```python
from build123d import *

# Parameters (mm, degrees)
F0_R     = 225
F1_DEPTH = 60


with BuildPart() as f1:
    # F0 (on Front) → F1 (new body)
    with BuildSketch(Plane.XZ):
        with BuildLine():
            ThreePointArc((228.965063, -4), (228.991266, -2.000076), (229, 0))
            ThreePointArc((229, 0), (228.991266, 2.000076), (228.965063, 4))
            ThreePointArc((228.965063, 4), (0, 229), (-228.965063, 4))
            ThreePointArc((-228.965063, 4), (-229, 0), (-228.965063, -4))
            ThreePointArc((-228.965063, -4), (0, -229), (228.965063, -4))
        make_face()
        Circle(F0_R, mode=Mode.SUBTRACT)
        with BuildLine():
            ThreePointArc((228.965063, 4), (228.991266, 2.000076), (229, 0))
            ThreePointArc((229, 0), (228.991266, -2.000076), (228.965063, -4))
            Line((228.965063, -4), (232.965486, -4))
            Line((232.965486, -4), (248.965063, -4))
            Line((248.965063, -4), (248.965063, 0))
            Line((248.965063, 0), (248.965063, 4))
            Line((248.965063, 4), (228.965063, 4))
        make_face()
        Polygon((232.965486, -4), (228.965063, -4), (225.022834, -274.970901), (-225.022834, -274.970901), (-228.965063, -4), (-232.965486, -4), (-228.965063, -278.970901), (228.965063, -278.970901), align=None)
        with BuildLine():
            ThreePointArc((-228.965063, -4), (-229, 0), (-228.965063, 4))
            Line((-228.965063, 4), (-248.965063, 4))
            Line((-248.965063, 4), (-248.965063, 0))
            Line((-248.965063, 0), (-248.965063, -4))
            Line((-248.965063, -4), (-232.965486, -4))
            Line((-232.965486, -4), (-228.965063, -4))
        make_face()
    extrude(amount=F1_DEPTH)


solid = f1.part
```
Design review of the part built by this model. Coordinates are the model's own, in mm. A direction names the side the tool comes from. Coordinates: 2 decimals unless noted, no trailing zeros. Order: outer loops, then holes, each group sorted by start corner. A loop starts at its lowest first (then second) coordinate and runs counter-clockwise, first axis right, second up. Notation, with made-up numbers: M -25.75,74.5 L -11.75,74.5 A21 ccw -11.75,105.5 Z; hole C -29,-26 d3. An arc over 180 degrees is marked long. Answer as a JSON object with one key per item and string values. Group by question number.
1) Add section C-C, the plane z = -146.5. Write out the cut boundary in (x, y).
2) Mouldability with a two-part tool opening along X and no side actions: class faces 1 (the flat face through (-239, -30, 4)), 2 (the cylindrical face through (-4.98, -29.58, -228.946)), 3 (the cylindrical face through (4.98, -29.58, 228.946)) as pulls with the +X half, pulls with the -X half, needs draft (parallel to the pull), parting line crosses it, or undercut.
3) For pin 1 (10 mm diameter, centred on x = -235.5, y = -30, fed in from +Z); pin 2 (2 mm diameter, centred on y = -29.5, z = 99.5, fed in from +X); pin 3 (12 mm diameter, centred on y = -42.5, z = -102.5, fed in from -X), all flat-tipped, find the tip position at first contact; note any pin that passes through.
4) Add section D-D, the plane x = -191. Write out the cut boundary in (y, z).
5) Wall thickness on L1, parallel to Z at x = -195, y = -8; L2, parallel to Z at x = -145, y = -52; L3, parallel to X at y = -15, z = -57.5: over which ranges is each line inside the solid? List them lowest first.
6) Tool access review of faces 4 (the flat face through (239, -30, 4)), 5 (the flat face through (3, -30, -274.971)), 6 (the flat face through (241, -30, -4)), 7 (the flat face through (-241, -30, -4)): name each direction out of +Z, -Z, +X, -X, +Y, -Y from which nothing blocks a thin tool from reaching the whole face with its end or side.
Computed values:
{
 "1": {"outline": "M -230.89,-60 L -226.89,-60 L -226.89,0 L -230.89,0 Z; M -176.01,-60 L -170.77,-60 L -170.77,0 L -176.01,0 Z; M 170.77,-60 L 176.01,-60 L 176.01,0 L 170.77,0 Z; M 226.89,-60 L 230.89,-60 L 230.89,0 L 226.89,0 Z"},
 "2": {"face 1": "needs draft", "face 2": "undercut", "face 3": "parting line crosses it"},
 "3": {"pin 1": "stops at z = 4", "pin 2": "stops at x = 206.73", "pin 3": "stops at x = -231.62"},
 "4": {"outline": "M -60,-278.97 L 0,-278.97 L 0,-274.97 L -60,-274.97 Z; M -60,-126.33 L 0,-126.33 L 0,-118.93 L -60,-118.93 Z; M -60,118.93 L 0,118.93 L 0,126.33 L -60,126.33 Z"},
 "5": {"L1": "z = -278.97 to -274.97, -120.07 to -112.25, 112.25 to 120.07", "L2": "z = -278.97 to -274.97, -177.25 to -172.05, 172.05 to 177.25", "L3": "x = -232.19 to -228.19, -221.66 to -217.53, 217.53 to 221.66, 228.19 to 232.19"},
 "6": {"face 4": "+Z, +X, +Y, -Y", "face 5": "+Y, -Y", "face 6": "-Z, +X, +Y, -Y", "face 7": "-Z, -X, +Y, -Y"}
}
